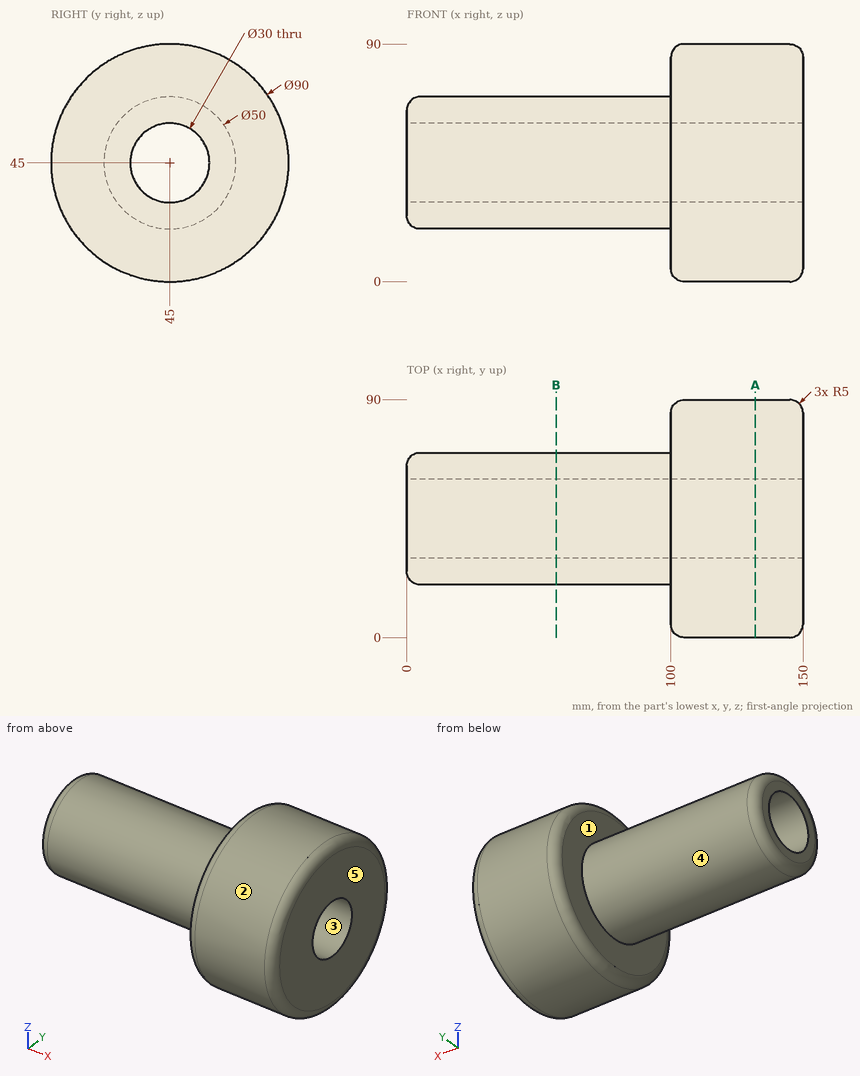
Study the drawing (mm; zero at the part's minimum x, y, z) and answer. A direction names the side the tool comes from. Coordinates: 2 decimals unless noted, no trailing zeros. Order: outer loops, then holes, each group sorted by start corner. A loop starts at its lowest first (then second) coordinate and runs counter-clockwise, first axis right, second up. Notation, with made-up numbers: (23.25, 50) -> (51.25, 50) arc R9 ccw to (51.25, 66) -> close; hole circle Ø7 at (86, 28.5). An arc over 180 degrees is marked (long way). Answer in a Markdown table with one row per item. Add a question column.
Item 1: Each of these flat-tipped pins is pushed along its axis until it touches: P1, Ø5, axis at y = 64, z = 42, coming from the -X side; P2, Ø8, axis at x = 47, y = 48.5, coming from the -Z side; P3, Ø24, axis at y = 45, z = 45, coming from the -X side; P4, Ø3, axis at x = 32, y = 21.5, coming from the +Z side. Where does it stop, or does it pass through?
Item 2: Find section B-B (x = 56.5). Write down the section's boundary in (y, z).
Item 3: Find section A-A (x = 132). Write down the section's boundary in (y, z).
Item 4: Which of the six approach directions +Z, -Z, +X, -X, +Y, -Y give full straight-line access (tool end or side, diameter ignored) to the marked faces 4 and 5?
Item 5: Determine the mould class of the marked faces 1, 2 and 3 for opening direction Y: +Y half, -Y half, draft (parallel to the pull), parting line (faces both ways), or undercut.
Item 6: Find the intervals of material crossed by L1, parallel to Z at x = 67, y = 45; L2, parallel to X at y = 37.5, z = 80; L3, parallel to Y at x = 130.5, z = 44, in increasing order. Write a range as from..to.
Result set:
| question | item | result |
|---|---|---|
| 1 | P1 | stops at x = 0 |
| 1 | P2 | stops at z = 20 |
| 1 | P3 | passes through |
| 1 | P4 | stops at z = 56.87 |
| 2 | outline | circle Ø50 at (45, 45); hole circle Ø30 at (45, 45) |
| 3 | outline | circle Ø90 at (45, 45); hole circle Ø30 at (45, 45) |
| 4 | face 4 | -X |
| 4 | face 5 | +Z, -Z, +X, +Y, -Y |
| 5 | face 1 | draft |
| 5 | face 2 | parting line |
| 5 | face 3 | undercut |
| 6 | L1 | z = 20..30, 60..70 |
| 6 | L2 | x = 100..150 |
| 6 | L3 | y = 0.01..30.03, 59.97..89.99 |
